Design review of the part built by this model. Coordinates are the model's own, in mm. A direction names the side the tool comes from. Round coordinates to 2 decimals unless told otherwise and drop trailing zeros. Write each loop counter-clockwise with the first axis right and the second up, starting at its lowest first coordinate (ties: lowest second). Pieces come first, ordered by that corner, then holes. Notation, with made-up numbers: M 63,53.5 L 68,53.5 A33 cw 68,81.5 Z; hole C -3,-7 d5. An arc over 180 degrees is marked long. Use CSV: the item, a comma, the result in double quotes.
from build123d import *

# Parameters (mm, degrees)
SKETCH1_R           = 46
SKETCH1_R_2         = 40
BOSS_EXTRUDE1_DEPTH = 4.7625
BOSS_EXTRUDE2_DEPTH = 4.7625
CIRPATTERN1_COUNT   = 4


with BuildPart() as part:
    # Sketch1 → Boss-Extrude1 (new body)
    with BuildSketch(Plane(origin=(0, 0, 0), x_dir=(1, 0, 0), z_dir=(0, 1, 0))):
        Circle(SKETCH1_R)
        Circle(SKETCH1_R_2, mode=Mode.SUBTRACT)
    extrude(amount=BOSS_EXTRUDE1_DEPTH)

    # Sketch2 → Boss-Extrude2 (add)
    with BuildSketch(Plane(origin=(0, 4.7625, 0), x_dir=(1, 0, 0), z_dir=(0, 1, 0))):
        with BuildLine():
            Line((-43.48562981, 15), (-50, 15))
            Line((-50, 15), (-50, -15))
            Line((-50, -15), (-43.48562981, -15))
            ThreePointArc((-43.48562981, -15), (-46, 0), (-43.48562981, 15))
        make_face()
    boss_extrude2 = extrude(amount=-BOSS_EXTRUDE2_DEPTH)

    # CirPattern1: Boss-Extrude2 ×4 about axis
    cirpattern1_axis = Axis((0, 0, 0), (0, 1, 0))
    for i in range(1, CIRPATTERN1_COUNT):
        add(boss_extrude2.rotate(cirpattern1_axis, i * 360 / CIRPATTERN1_COUNT))


solid = part.part
1) For pin 1 Ø1 at (y, z) = (1.5, 30.5) entering from -X; pin 2 Ø1.4 at (x, y) = (46.5, 3.5) entering from -Z, all flat-tipped, find the tip position at first contact; note any pin that passes through.
Answers:
pin 1,"x = -34.87"
pin 2,"z = -15"
2) Add section B-B on x = 0. Write out the cut boundary in (y, z).
Answers:
outline,"M 0,-50 L 4.76,-50 L 4.76,-40 L 0,-40 Z; M 0,40 L 4.76,40 L 4.76,50 L 0,50 Z"
3) Add section A-A on z = 0. Write out the cut boundary in (x, y), then the cut area to 4 significant figures.
Answers:
outline,"M -50,0 L -40,0 L -40,4.76 L -50,4.76 Z; M 40,0 L 50,0 L 50,4.76 L 40,4.76 Z"
area,"95.25 mm²"
4) The part is to be moulded in two halves that separate along X. For faces 6 (the face through (15, 2, -47)), 7 (the face through (-8.67, 2.35, 39.05)), 8 (the face through (0, 2, -50)), 9 (the face through (-15, 2, -47)), say which applies: released by +X, released by -X, zero draft, split by the parting line, or undercut.
Answers:
face 6,"released by +X"
face 7,"undercut"
face 8,"zero draft"
face 9,"released by -X"
5) Add section C-C on y = 2.95. Write out the cut boundary in (x, z), then the cut area to 3 significant figures.
Answers:
outline,"M -50,-15 L -43.49,-15 A46 ccw -15,-43.49 L -15,-50 L 15,-50 L 15,-43.49 A46 ccw 43.49,-15 L 50,-15 L 50,15 L 43.49,15 A46 ccw 15,43.49 L 15,50 L -15,50 L -15,43.49 A46 ccw -43.49,15 L -50,15 Z; hole C 0,0 d80"
area,"2,200 mm²"
6) Machinability: for faces 1 (the face through (-47, 2, -15)), 2 (the face through (47, 2, 15)), 3 (the face through (0, 2, 50)), 4 (the face through (47, 2, -15)), 5 (the face through (-15, 2, 47)), which of the approach directions +Z, -Z, +X, -X, +Y, -Y give a long, thin tool a straight path to every point of the face, cutting with its end or side? Answer none if there is none.
Answers:
face 1,"-Z, -X, +Y, -Y"
face 2,"+Z, +X, +Y, -Y"
face 3,"+Z, +X, -X, +Y, -Y"
face 4,"-Z, +X, +Y, -Y"
face 5,"+Z, -X, +Y, -Y"
7) Wall thickness on line 1 along Z through (x, y) = (0, 1.15); line 2 along X through (y, z) = (1.35, -9): over which ranges is each line inside the solid? List them lowest first. Write a range as [from, to].
Answers:
line 1,"[-50, -40], [40, 50]"
line 2,"[-50, -38.97], [38.97, 50]"
